Work out the finished part from the listing and answer in its coordinate system (mm). Face numbers are marked on the shaded views. A direction names the side the tool comes from. Coordinates: 2 decimals unless noted, no trailing zeros. Write each loop counter-clockwise with the first axis right and the second up, starting at its lowest first coordinate (ties: lowest second). Pieces come first, ordered by that corner, then holes. Notation, with made-up numbers: M 44.5,17 L 69.5,17 A20 cw 69.5,23 Z; hole C -1,57.25 d9. An arc over 180 degrees is marked long. Answer as CSV lines item,"result". Start each with the question number.
(1) A cutting plane is placed at A-A on x = -11.43. Give the vertices of the cut face in (y, z).
(2) For the marked faces 1, 2, 3 and 4, determine the directions among +Z, -Z, +X, -X, +Y, -Y from which every point of the face is accessible in a straight line to the end or side of a thin tool.
(3) Find the intervals of material crossed by L1, parallel to Z at x = -23.5, y = -31; L2, parallel to Y at x = -11.43, z = 74; L3, parallel to Y at x = 9.5, z = 97, in increasing order. Write a range as [from, to].
(4) A cutting plane is placed at B-B on z = 13. Give the vertices of the cut face in (x, y), then the cut area to 3 significant figures.
(5) The mould has two halves that part along Y. Classify the marked faces 5, 6 and 7: released by +Y, released by -Y, zero draft, split by the parting line, or undercut.
(6) Flat-ended cylindrical pins translate along their axes: P1, Ø4, axis at x = 5.5, z = 42.5, coming from the -Y side; P2, Ø1.9, axis at x = -3, z = 99.5, coming from the +Y side; P3, Ø12, axis at y = 8, z = 29.5, coming from the +X side. Find the tip coordinate at first contact, or state that the pin passes through.
(7) A cutting plane is placed at D-D on x = -22.5. Give the vertices of the cut face in (y, z).
(8) A cutting plane is placed at C-C on y = 37.5. Give the vertices of the cut face in (x, z).
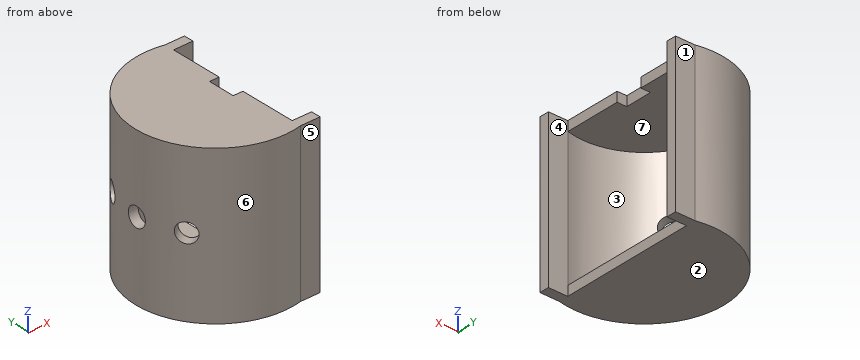
from build123d import *

# Parameters (mm, degrees)
BOSS_EXTRUDE1_DEPTH                      = 101.6
SHELL1_T                                 = -6.35
SKETCH3_W                                = 6.35
SKETCH3_H                                = 17.78
CUT_EXTRUDE1_DEPTH                       = 6.35
SKETCH4_W                                = 12.7
SKETCH4_H                                = 6.35
BOSS_EXTRUDE2_DEPTH                      = 101.6
SKETCH6_W                                = 12.7
SKETCH6_H                                = 6.35
BOSS_EXTRUDE3_DEPTH                      = 101.6
F_1_2_0_5_DIAMETER_HOLE1_D               = 12.7
F_1_2_0_5_DIAMETER_HOLE1_DEPTH           = 7.62
F_1_2_0_5_DIAMETER_HOLE1_TIP             = 3.815464931
F_1_2_0_5_DIAMETER_HOLE1_ON_FACE_2_D     = 12.7
F_1_2_0_5_DIAMETER_HOLE1_ON_FACE_2_DEPTH = 7.62
F_1_2_0_5_DIAMETER_HOLE1_ON_FACE_2_TIP   = 3.815464931
F_1_2_0_5_DIAMETER_HOLE1_ON_FACE_3_D     = 12.7
F_1_2_0_5_DIAMETER_HOLE1_ON_FACE_3_DEPTH = 7.62
F_1_2_0_5_DIAMETER_HOLE1_ON_FACE_3_TIP   = 3.815464931


with BuildPart() as part:
    # Sketch2 → Boss-Extrude1 (new body)
    with BuildSketch(Plane.XY):
        with BuildLine():
            Line((0, -50.8), (0, 0))
            Line((0, 0), (0, 50.8))
            ThreePointArc((0, 50.8), (-63.5, 0), (0, -50.8))
        make_face()
    extrude(amount=BOSS_EXTRUDE1_DEPTH)

    # Shell1
    shell1_openings = [part.faces().sort_by_distance(p)[0] for p in [
        (0, 0, 50.8),
    ]]
    offset(amount=SHELL1_T, openings=shell1_openings)

    # Sketch3 → Cut-Extrude1 (cut)
    with BuildSketch(Plane.XY.offset(101.6)):
        with Locations((-3.175, 1.38458233)):
            Rectangle(SKETCH3_W, SKETCH3_H)
    extrude(amount=-CUT_EXTRUDE1_DEPTH, mode=Mode.SUBTRACT)

    # Sketch4 → Boss-Extrude2 (add)
    with BuildSketch(Plane.XY.offset(101.6)):
        with Locations((6.35, 47.625)):
            Rectangle(SKETCH4_W, SKETCH4_H)
    extrude(amount=-BOSS_EXTRUDE2_DEPTH)

    # Sketch6 → Boss-Extrude3 (add)
    with BuildSketch(Plane.XY.offset(101.6)):
        with Locations((6.35, -47.625)):
            Rectangle(SKETCH6_W, SKETCH6_H)
    extrude(amount=-BOSS_EXTRUDE3_DEPTH)

    # 1/2 (0.5) Diameter Hole1
    with Locations(Plane(origin=(-63.499461497, -0.236811011, 51.161863275), x_dir=(0.004547935689, -0.999989658087, 0), z_dir=(-0.999989658087, -0.004547935689, 0))):
        with Locations((0, 0)):
            Hole(F_1_2_0_5_DIAMETER_HOLE1_D / 2, depth=F_1_2_0_5_DIAMETER_HOLE1_DEPTH)
            with Locations((0, 0, -(F_1_2_0_5_DIAMETER_HOLE1_DEPTH + F_1_2_0_5_DIAMETER_HOLE1_TIP / 2))):  # 118° drill point
                Cone(0, F_1_2_0_5_DIAMETER_HOLE1_D / 2, F_1_2_0_5_DIAMETER_HOLE1_TIP, mode=Mode.SUBTRACT)

    # 1/2 (0.5) Diameter Hole1 on face 2
    with Locations(Plane(origin=(-55.14102988, -28.295419537, 51.457217049), x_dir=(0.543410902455, -0.839466849312, 0), z_dir=(-0.839466849312, -0.543410902455, 0))):
        with Locations((0, 0)):
            Hole(F_1_2_0_5_DIAMETER_HOLE1_ON_FACE_2_D / 2, depth=F_1_2_0_5_DIAMETER_HOLE1_ON_FACE_2_DEPTH)
            with Locations((0, 0, -(F_1_2_0_5_DIAMETER_HOLE1_ON_FACE_2_DEPTH + F_1_2_0_5_DIAMETER_HOLE1_ON_FACE_2_TIP / 2))):  # 118° drill point
                Cone(0, F_1_2_0_5_DIAMETER_HOLE1_ON_FACE_2_D / 2, F_1_2_0_5_DIAMETER_HOLE1_ON_FACE_2_TIP, mode=Mode.SUBTRACT)

    # 1/2 (0.5) Diameter Hole1 on face 3
    with Locations(Plane(origin=(-56.343520967, 26.345028645, 50.866509501), x_dir=(-0.505954201442, -0.862560343422, 0), z_dir=(-0.862560343422, 0.505954201442, 0))):
        with Locations((0, 0)):
            Hole(F_1_2_0_5_DIAMETER_HOLE1_ON_FACE_3_D / 2, depth=F_1_2_0_5_DIAMETER_HOLE1_ON_FACE_3_DEPTH)
            with Locations((0, 0, -(F_1_2_0_5_DIAMETER_HOLE1_ON_FACE_3_DEPTH + F_1_2_0_5_DIAMETER_HOLE1_ON_FACE_3_TIP / 2))):  # 118° drill point
                Cone(0, F_1_2_0_5_DIAMETER_HOLE1_ON_FACE_3_D / 2, F_1_2_0_5_DIAMETER_HOLE1_ON_FACE_3_TIP, mode=Mode.SUBTRACT)


solid = part.part
Here are the results:
1,outline,"M -52.07,0 L 52.07,0 L 52.07,101.6 L -52.07,101.6 Z; hole M -45.72,6.35 L 45.72,6.35 L 45.72,95.25 L -45.72,95.25 Z"
2,face 1,"+Z, -Z, +X, +Y"
2,face 2,"-Z, +X, -X, +Y, -Y"
2,face 3,"none"
2,face 4,"+Z, -Z, +X"
3,L1,"z = [0, 6.35], [95.25, 101.6]"
3,L2,"y = [-52.07, -45.72], [45.72, 52.07]"
3,L3,"y = [-50.8, -44.45], [44.45, 50.8]"
4,outline,"M 0,-50.8 L 12.7,-50.8 L 12.7,-44.45 L 0,-44.45 L 0,-44.27 A45.72 cw long 0,44.27 L 0,44.45 L 12.7,44.45 L 12.7,50.8 L 0,50.8 A52.07 ccw long Z"
4,area,"1,280 mm^2"
5,face 5,"released by -Y"
5,face 6,"split by the parting line"
5,face 7,"undercut"
6,P1,"stops at y = -50.8"
6,P2,"stops at y = 51.53"
6,P3,"stops at x = -54.95"
7,outline,"M -50.88,0 L 50.88,0 L 50.88,101.6 L -50.88,101.6 Z; hole M -44.36,6.35 L 44.36,6.35 L 44.36,95.25 L -44.36,95.25 Z"
8,outline,"M -47.56,0 L 0,0 L 0,6.35 L -37.58,6.35 L -37.58,95.25 L 0,95.25 L 0,101.6 L -47.56,101.6 Z"
